The model under review builds one solid part; all positions refer to its coordinate system, in mm. Round coordinates to 2 decimals unless told otherwise and drop trailing zeros. Write each loop counter-clockwise with the first axis right and the second up, starting at its lowest first coordinate (ties: lowest second). Pieces come first, ordered by that corner, then holes. Notation, with made-up numbers: (22, 81.5) - (64, 81.5) arc R31 ccw to (64, 108.5) - close; hole circle Ø6 at (48.25, 3). An arc over 180 degrees is marked (long way). Use one line per item in the form item = value.
from build123d import *

# Parameters (mm, degrees)
SKETCH2_W           = 200
SKETCH2_H           = 100
SKETCH2_W_2         = 45
SKETCH2_H_2         = 45
BOSS_EXTRUDE1_DEPTH = 5
FILLET2_R           = 1


with BuildPart() as part:
    # Sketch2 → Boss-Extrude1 (new body)
    with BuildSketch(Plane.XY):
        with Locations((0, 50)):
            Rectangle(SKETCH2_W, SKETCH2_H)
        with Locations((-75, 75)):
            Rectangle(SKETCH2_W_2, SKETCH2_H_2, mode=Mode.SUBTRACT)
        with Locations((-25, 75)):
            Rectangle(SKETCH2_W_2, SKETCH2_H_2, mode=Mode.SUBTRACT)
        with Locations((75, 25)):
            Rectangle(SKETCH2_W_2, SKETCH2_H_2, mode=Mode.SUBTRACT)
        with Locations((25, 75)):
            Rectangle(SKETCH2_W_2, SKETCH2_H_2, mode=Mode.SUBTRACT)
        with Locations((75, 75)):
            Rectangle(SKETCH2_W_2, SKETCH2_H_2, mode=Mode.SUBTRACT)
        with Locations((-75, 25)):
            Rectangle(SKETCH2_W_2, SKETCH2_H_2, mode=Mode.SUBTRACT)
        with Locations((-25, 25)):
            Rectangle(SKETCH2_W_2, SKETCH2_H_2, mode=Mode.SUBTRACT)
        with Locations((25, 25)):
            Rectangle(SKETCH2_W_2, SKETCH2_H_2, mode=Mode.SUBTRACT)
    extrude(amount=BOSS_EXTRUDE1_DEPTH)

    # Fillet2
    fillet2_edges = [part.edges().sort_by_distance(p)[0] for p in [
        (-75, 97.5, 5),
        (-97.5, 75, 5),
        (-75, 52.5, 5),
        (-52.5, 75, 5),
        (-100, 50, 5),
        (-25, 47.5, 5),
        (0, 0, 5),
        (-47.5, 25, 5),
        (-25, 2.5, 5),
        (-2.5, 25, 5),
        (25, 47.5, 5),
        (2.5, 25, 5),
        (25, 2.5, 5),
        (47.5, 25, 5),
        (75, 47.5, 5),
        (52.5, 25, 5),
        (75, 2.5, 5),
        (97.5, 25, 5),
        (100, 50, 5),
        (-25, 97.5, 5),
        (-47.5, 75, 5),
        (-25, 52.5, 5),
        (-2.5, 75, 5),
        (47.5, 75, 5),
        (25, 97.5, 5),
        (2.5, 75, 5),
        (25, 52.5, 5),
        (97.5, 75, 5),
        (75, 97.5, 5),
        (52.5, 75, 5),
        (75, 52.5, 5),
        (0, 100, 5),
        (-52.5, 25, 5),
        (-75, 47.5, 5),
        (-97.5, 25, 5),
        (-75, 2.5, 5),
    ]]
    fillet(fillet2_edges, radius=FILLET2_R)


solid = part.part
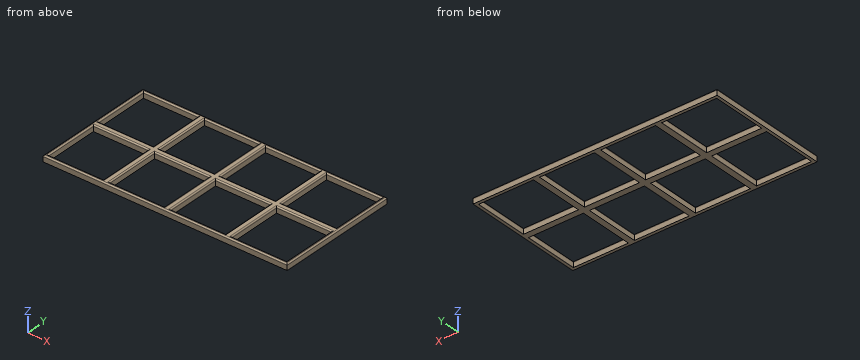
(1) To check wall thickness, follow L1, parallel to Y at x = -55.5, z = 4.15; L2, parallel to X at y = 91, z = 2.2; L3, parallel to X at y = 47.5, z = 4.55. State the ranges of each line that lie inside material, in increasing order.
Geometry results:
L1 = 0.01 to 2.49, 47.51 to 52.49, 97.51 to 99.99
L2 = -100 to -97.5, -52.5 to -47.5, -2.5 to 2.5, 47.5 to 52.5, 97.5 to 100
L3 = -99.84 to -97.66, -52.34 to -47.66, -2.34 to 2.34, 47.66 to 52.34, 97.66 to 99.84
(2) Add section B-B on x = -83.5. Write out the cut boundary in (y, z), then the cut area to 3 significant figures.
Geometry results:
outline = (0, 0) - (2.5, 0) - (2.5, 4) arc R1 ccw to (1.5, 5) - (1, 5) arc R1 ccw to (0, 4) - close; (47.5, 0) - (52.5, 0) - (52.5, 4) arc R1 ccw to (51.5, 5) - (48.5, 5) arc R1 ccw to (47.5, 4) - close; (97.5, 0) - (100, 0) - (100, 4) arc R1 ccw to (99, 5) - (98.5, 5) arc R1 ccw to (97.5, 4) - close
area = 48.7 mm2
(3) Add section A-A on y = 68.5. Count the separate pieces of the cut face and the enclosed holes in it, then the cut area to 3 significant figures.
Geometry results:
separate_pieces = 5
enclosed_holes = 0
area = 97.9 mm2
